```python
from build123d import *

# Parameters (mm, degrees)
SKETCH2_R           = 4
CUT_EXTRUDE1_DEPTH  = 10
SKETCH5_W           = 110
SKETCH5_H           = 5
BOSS_EXTRUDE1_DEPTH = 13
SKETCH6_R           = 9
CUT_EXTRUDE2_DEPTH  = 13
CUT_EXTRUDE3_DEPTH  = 10


with BuildPart() as part:
    # Sweep1: sweep along a path in Sketch1
    with BuildLine(Plane(origin=(0, 0, 0), x_dir=(1, 0, 0), z_dir=(0, 1, 0))) as sweep1_path:
        Line((52.389202821, -40.03089611), (-0.272615345, -6.763487127))
        ThreePointArc((-0.272615345, -6.763487127), (-3.006458548, -3.861287171), (-4, 0))
    # Sketch2 → Sweep1 (sweep)
    with BuildSketch(Plane.XY):
        with Locations((-4, 0)):
            Circle(SKETCH2_R)
    sweep1 = sweep(path=sweep1_path.line)

    # Sketch4 → Cut-Extrude1 (cut, symmetric)
    with BuildSketch(Plane(origin=(0, 0, 0), x_dir=(1, 0, 0), z_dir=(0, 1, 0))):
        Polygon((44, -35), (34.597308022, -35), (44, -46.531698577), (57.177061071, -46.531698577), (57.177061071, -30), (44, -30), align=None)
    cut_extrude1 = extrude(amount=CUT_EXTRUDE1_DEPTH, both=True, mode=Mode.SUBTRACT)

    # Sketch5 → Boss-Extrude1 (add, symmetric)
    with BuildSketch(Plane(origin=(0, 0, 0), x_dir=(1, 0, 0), z_dir=(0, 1, 0))):
        with Locations((99, -32.5)):
            Rectangle(SKETCH5_W, SKETCH5_H)
    boss_extrude1 = extrude(amount=BOSS_EXTRUDE1_DEPTH, both=True)

    # Sketch6 → Cut-Extrude2 (cut, symmetric)
    with BuildSketch(Plane.XY.offset(35)):
        with Locations((141, 0)):
            Circle(SKETCH6_R)
        with BuildLine():
            Line((53, 13), (52.778372403, 14.264161609))
            Line((52.778372403, 14.264161609), (42.606717514, 14.264161609))
            Line((42.606717514, 14.264161609), (42.848324519, 6.72602307))
            Line((42.848324519, 6.72602307), (44, 4))
            ThreePointArc((44, 4), (46.636038969, 10.363961031), (53, 13))
        make_face()
    cut_extrude2 = extrude(amount=CUT_EXTRUDE2_DEPTH, both=True, mode=Mode.SUBTRACT)

    # Sketch7 → Cut-Extrude3 (cut)
    with BuildSketch(Plane.XY.offset(35)):
        with BuildLine():
            Line((44, -13), (53, -13))
            ThreePointArc((53, -13), (46.636038969, -10.363961031), (44, -4))
            Line((44, -4), (44, -13))
        make_face()
        with BuildLine():
            ThreePointArc((154, 1.44e-07), (150.192388206, -9.192388104), (141, -13))
            Line((141, -13), (154, -13))
            Line((154, -13), (154, 1.44e-07))
        make_face()
        with BuildLine():
            ThreePointArc((141, 13), (150.192388104, 9.192388206), (154, 1.44e-07))
            Line((154, 1.44e-07), (154, 13))
            Line((154, 13), (141, 13))
        make_face()
    cut_extrude3 = extrude(amount=-CUT_EXTRUDE3_DEPTH, mode=Mode.SUBTRACT)

    # Mirror1: Sweep1, Cut-Extrude1, Boss-Extrude1, Cut-Extrude2, Cut-Extrude3 across plane
    add(sweep1.mirror(Plane(origin=(-4, 0, 0), x_dir=(1, 0, 0), z_dir=(0, 0, 1))))
    add(cut_extrude1.mirror(Plane(origin=(-4, 0, 0), x_dir=(1, 0, 0), z_dir=(0, 0, 1))), mode=Mode.SUBTRACT)
    add(boss_extrude1.mirror(Plane(origin=(-4, 0, 0), x_dir=(1, 0, 0), z_dir=(0, 0, 1))))
    add(cut_extrude2.mirror(Plane(origin=(-4, 0, 0), x_dir=(1, 0, 0), z_dir=(0, 0, 1))), mode=Mode.SUBTRACT)
    add(cut_extrude3.mirror(Plane(origin=(-4, 0, 0), x_dir=(1, 0, 0), z_dir=(0, 0, 1))), mode=Mode.SUBTRACT)


solid = part.part
```
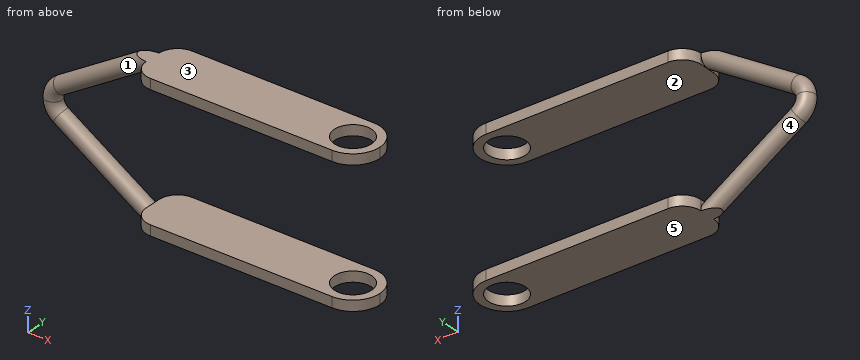
Model file for the job. Use its own axes, mm. Face numbers are marked on the shaded views. A direction names the side the tool comes from. Coordinates: 2 decimals unless noted, no trailing zeros. Write each loop counter-clockwise with the first axis right and the second up, starting at its lowest first coordinate (ties: lowest second). Pieces come first, ordered by that corner, then holes. Notation, with made-up numbers: (38.25, 41) - (61.25, 41) arc R25 ccw to (61.25, 58) - close; hole circle Ø4 at (85.25, -32.75). An arc over 180 degrees is marked (long way). Use a Markdown table: item, result. Add a question column.
Item 1: Two-plate mould, pull along Z, no slides. Class the marked faces 3, 4 and 5: pulls with the +Z half, pulls with the -Z half, needs draft (parallel to the pull), parting line crosses it, or undercut.
Item 2: Band-saw the part on B-B, the plane y = 10.75. Write the cut outline in (x, z).
Item 3: Band-saw the part on A-A, the plane x = 55.5. Write the cut outline in (y, z).
Item 4: Drop flat-ended pins along their axis: pin 1 (1.2 mm diameter, centred on y = 2.5, z = -31.5, fed in from -X); pin 2 (1.2 mm diameter, centred on y = -1, z = 33, fed in from -X); pin 3 (4.5 mm diameter, centred on y = 2.5, z = 31.5, fed in from -X). Give the stop position or say it passes through.
Item 5: 3-axis set-ups, long thin cutter, end or side, ignore diameter. For the marked faces 1 and 2: which of +Z, -Z, +X, -X, +Y, -Y reach the whole face in a straight line?
Item 6: Drill centre lines: line 1 along Z through (x, y) = (60, 4.5); line 2 along Y through (x, z) = (141, 32.45); line 3 along Z through (x, y) = (6, 2.5). Where is each one in solid material? Low to high.
A:
| question | item | result |
|---|---|---|
| 1 | face 3 | pulls with the +Z half |
| 1 | face 4 | undercut |
| 1 | face 5 | pulls with the -Z half |
| 2 | outline | (47.05, -35) - (148.31, -35) - (148.31, -30) - (47.05, -30) - close; (47.05, 30) - (148.31, 30) - (148.31, 35) - (47.05, 35) - close |
| 3 | outline | (-13, -35) - (13, -35) - (13, -30) - (-13, -30) - close; (-13, 30) - (13, 30) - (13, 35) - (-13, 35) - close |
| 4 | pin 1 | stops at x = 31.8 |
| 4 | pin 2 | stops at x = 33.02 |
| 4 | pin 3 | stops at x = 28.75 |
| 5 | face 1 | none |
| 5 | face 2 | +X, +Y, -Y |
| 6 | line 1 | z = -35 to -30, 30 to 35 |
| 6 | line 2 | y = -13 to -9, 9 to 13 |
| 6 | line 3 | z = -14.42 to -7.03, 7.03 to 14.42 |
